Part print with two shaded views. Sizes in mm from the minimum x, y, z corner. A direction names the side the tool comes from. Round coordinates to 2 decimals unless told otherwise and drop trailing zeros. Order: outer loops, then holes, each group sorted by start corner. A loop starts at its lowest first (then second) coordinate and runs counter-clockwise, first axis right, second up. Notation, with made-up numbers: (-22, 74) - (3, 74) arc R18 ccw to (3, 102) - close; hole circle Ø8 at (0.5, 44). An arc over 180 degrees is marked (long way). Answer as CSV lines item,"result". Start each with the question number.
1. 3-axis set-ups, long thin cutter, end or side, ignore diameter. For the marked faces 1 and 2: which of +Z, -Z, +X, -X, +Y, -Y reach the whole face in a straight line?
2. Band-saw the part on D-D on z = 19.5. List the corners of the cut face in (x, y).
3. Band-saw the part on B-B on y = 27. List the corners of the cut face in (x, z).
4. Band-saw the part on A-A on z = 12.5. List the corners of the cut face in (x, y).
5. Pin check, flat tips, straight feed: pin 1 Ø4 at (x, z) = (31, 22) entering from +Y; pin 2 Ø5 at (y, z) = (27, 27.5) entering from +X; pin 3 Ø1.5 at (x, z) = (11.5, 25) entering from +Y; pin 4 Ø6 at (x, z) = (27.5, 20) entering from -Y. Stop position of each tip, or through.
6. Wall check: line 1 along Z through (x, y) = (27, 2.75); line 2 along Y through (x, z) = (38, 8.5). Give the ranges that are in metal, low to high. Write a range as [from, to].
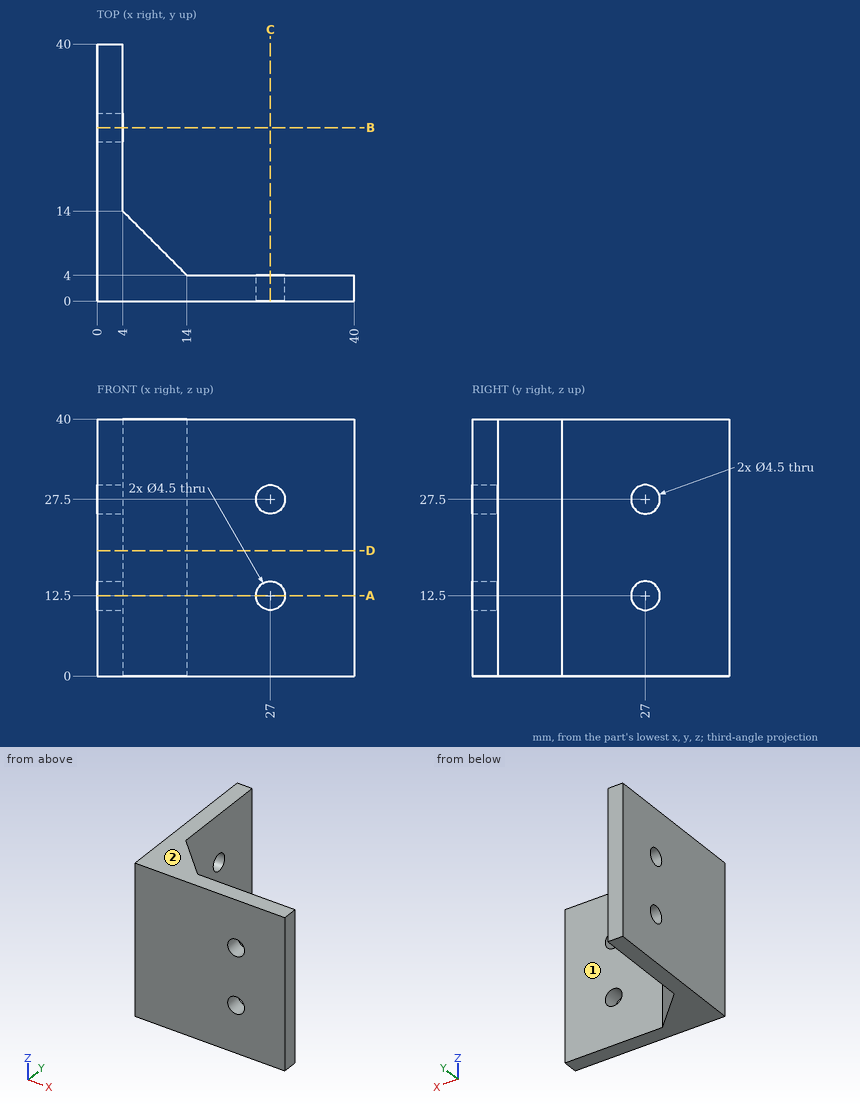
Reply:
1,face 1,"+Z, -Z, +X, +Y"
1,face 2,"+Z, +X, -X, +Y, -Y"
2,outline,"(0, 0) - (40, 0) - (40, 4) - (14, 4) - (4, 14) - (4, 40) - (0, 40) - close"
3,outline,"(0, 0) - (4, 0) - (4, 10.25) - (0, 10.25) - close; (0, 14.75) - (4, 14.75) - (4, 25.25) - (0, 25.25) - close; (0, 29.75) - (4, 29.75) - (4, 40) - (0, 40) - close"
4,outline,"(0, 0) - (24.75, 0) - (24.75, 4) - (14, 4) - (4, 14) - (4, 24.75) - (0, 24.75) - close; (0, 29.25) - (4, 29.25) - (4, 40) - (0, 40) - close; (29.25, 0) - (40, 0) - (40, 4) - (29.25, 4) - close"
5,pin 1,"stops at y = 4"
5,pin 2,"stops at x = 4"
5,pin 3,"stops at y = 7.25"
5,pin 4,"stops at y = 0"
6,line 1,"z = [0, 10.25], [14.75, 25.25], [29.75, 40]"
6,line 2,"y = [0, 4]"
